Here's the drawing with two shaded views (mm, measured from the low corner). I have some questions. A direction names the side the tool comes from. Round coordinates to 2 decimals unless told otherwise and drop trailing zeros. Loops run counter-clockwise (first coordinate to the right, second up) from the corner with the lowest first, then second, coordinate; pieces in that order, holes last. Notation, with made-up numbers: M 68,-18.75 L 111,-18.75 A6 cw 111,-13.75 Z; hole C 48.25,-2 d9. An arc over 180 degrees is marked long. Write each question's results on one line, items separated by ' | '. Start each with the question number.
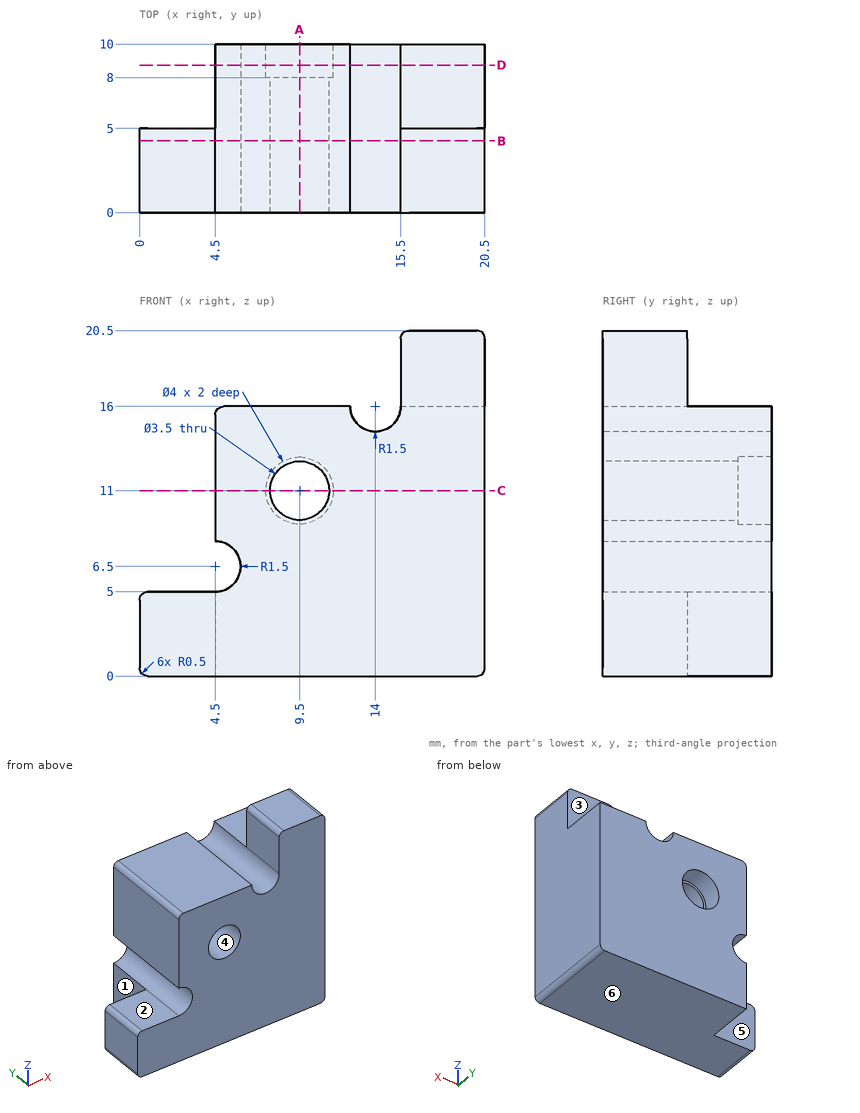
Item 1: I'm going to push flat-ended pins straight in: pin 1 (6 mm diameter, centred on x = 9, y = 5.5, fed in from +Z); pin 2 (4 mm diameter, centred on y = 5, z = 12, fed in from -X); pin 3 (4 mm diameter, centred on x = 9.5, z = 11, fed in from -Y); pin 4 (1.3 mm diameter, centred on x = 19, z = 17.5, fed in from +Y). Where does each tip first touch, or does it pass through?
Item 2: If we mould it in two halves opening along Z, with no side actions, what happens to the marked faces 4, 5 and 6? For each: released by +Z, released by -Z, zero draft, split by the parting line, or undercut.
Item 3: If we section it at B-B on y = 4.25: Please give me the cut outline in (x, z), and give its area (3 significant figures).
Item 4: If we section it at D-D on y = 8.75: Please give me the cut outline in (x, z), and give its area (3 significant figures).
Item 5: Which directions (+Z, -Z, +X, -X, +Y, -Y) give clear straight access to the entire face, cutting with the end or side of a thin tool? Please do the marked faces 1, 2 and 3.
Item 6: If we section it at A-A on x = 9.5: Please give me the cut outline in (y, z).
Item 7: If we section it at C-C on z = 11: Please give me the cut outline in (x, y), and give its area (3 significant figures).
Item 8: I need wall thicknesses on L1, parallel to X at y = 3.75, z = 11; L2, parallel to X at y = 8.65, z = 11; L3, parallel to Z at x = 7.5, y = 7.5. Which ranges of each line are inside material? Lowest first, please.
Numbers:
1) pin 1: z = 16 | pin 2: x = 4.5 | pin 3: y = 0 | pin 4: y = 5
2) face 4: undercut | face 5: zero draft | face 6: released by -Z
3) outline: M 0,0.5 A0.5 ccw 0.5,0 L 20,0 A0.5 ccw 20.5,0.5 L 20.5,20 A0.5 ccw 20,20.5 L 16,20.5 A0.5 ccw 15.5,20 L 15.5,16 A1.5 cw 12.5,16 L 5,16 A0.5 ccw 4.5,15.5 L 4.5,8 A1.5 cw 4.5,5 L 0.5,5 A0.5 ccw 0,4.5 Z; hole C 9.5,11 d3.5 | area: 284 mm²
4) outline: M 4.5,0 L 20,0 A0.5 ccw 20.5,0.5 L 20.5,16 L 15.5,16 A1.5 cw 12.5,16 L 5,16 A0.5 ccw 4.5,15.5 L 4.5,8 A1.5 cw 4.5,5 Z; hole C 9.5,11 d4 | area: 236 mm²
5) face 1: +Z, -Z, -X, +Y | face 2: +Z, -X, +Y, -Y | face 3: +Z, +X, -X, +Y
6) outline: M 0,0 L 10,0 L 10,9 L 8,9 L 8,9.25 L 0,9.25 Z; M 0,12.75 L 8,12.75 L 8,13 L 10,13 L 10,16 L 0,16 Z
7) outline: M 4.5,0 L 7.75,0 L 7.75,8 L 7.5,8 L 7.5,10 L 4.5,10 Z; M 11.25,0 L 20.5,0 L 20.5,10 L 11.5,10 L 11.5,8 L 11.25,8 Z | area: 124 mm²
8) L1: 4.5 to 7.75, 11.25 to 20.5 | L2: 4.5 to 7.5, 11.5 to 20.5 | L3: 0 to 16
